from build123d import *

# Parameters (mm, degrees)
SKETCH_1_R      = 1.1
SKETCH_1_R_2    = 1.6
SKETCH_1_R_3    = 15
EXTRUDE_1_DEPTH = 4


with BuildPart() as part:
    # 草图1 → 凸台-拉伸1 (new body)
    with BuildSketch(Plane(origin=(0, 0, 0), x_dir=(1, 0, 0), z_dir=(0, 1, 0))):
        with BuildLine():
            Line((-54, 60), (54, 60))
            ThreePointArc((54, 60), (58.242640687, 58.242640687), (60, 54))
            Line((60, 54), (60, -54))
            ThreePointArc((60, -54), (58.242640687, -58.242640687), (54, -60))
            Line((54, -60), (-54, -60))
            ThreePointArc((-54, -60), (-58.242640687, -58.242640687), (-60, -54))
            Line((-60, -54), (-60, 54))
            ThreePointArc((-60, 54), (-58.242640687, 58.242640687), (-54, 60))
        make_face()
        with Locations(Location((0, 18.6, 0), (0, 0, 270))):
            Circle(SKETCH_1_R, mode=Mode.SUBTRACT)
        with Locations(Location((8.8, -18.6, 0), (0, 0, 270))):
            Circle(SKETCH_1_R, mode=Mode.SUBTRACT)
        with Locations(Location((-8.8, -18.6, 0), (0, 0, 270))):
            Circle(SKETCH_1_R, mode=Mode.SUBTRACT)
        with Locations(Location((-21, 25, 0), (0, 0, 270))):
            Circle(SKETCH_1_R_2, mode=Mode.SUBTRACT)
        with Locations(Location((21, 25, 0), (0, 0, 90))):
            Circle(SKETCH_1_R_2, mode=Mode.SUBTRACT)
        with Locations(Location((21, -25, 0), (0, 0, 270))):
            Circle(SKETCH_1_R_2, mode=Mode.SUBTRACT)
        with Locations(Location((-21, -25, 0), (0, 0, 90))):
            Circle(SKETCH_1_R_2, mode=Mode.SUBTRACT)
        with Locations(Location((-56.25, 50, 0), (0, 0, 270))):
            Circle(SKETCH_1_R_2, mode=Mode.SUBTRACT)
        with Locations(Location((-44.25, 50, 0), (0, 0, 270))):
            Circle(SKETCH_1_R_2, mode=Mode.SUBTRACT)
        with Locations(Location((-44.25, 22, 0), (0, 0, 270))):
            Circle(SKETCH_1_R_2, mode=Mode.SUBTRACT)
        with Locations(Location((-56.25, 22, 0), (0, 0, 270))):
            Circle(SKETCH_1_R_2, mode=Mode.SUBTRACT)
        with Locations(Location((56.25, 22, 0), (0, 0, 270))):
            Circle(SKETCH_1_R_2, mode=Mode.SUBTRACT)
        with Locations(Location((44.25, 22, 0), (0, 0, 270))):
            Circle(SKETCH_1_R_2, mode=Mode.SUBTRACT)
        with Locations(Location((44.25, 50, 0), (0, 0, 270))):
            Circle(SKETCH_1_R_2, mode=Mode.SUBTRACT)
        with Locations(Location((56.25, 50, 0), (0, 0, 270))):
            Circle(SKETCH_1_R_2, mode=Mode.SUBTRACT)
        with Locations(Location((56.25, -50, 0), (0, 0, 270))):
            Circle(SKETCH_1_R_2, mode=Mode.SUBTRACT)
        with Locations(Location((44.25, -50, 0), (0, 0, 270))):
            Circle(SKETCH_1_R_2, mode=Mode.SUBTRACT)
        with Locations(Location((44.25, -22, 0), (0, 0, 270))):
            Circle(SKETCH_1_R_2, mode=Mode.SUBTRACT)
        with Locations(Location((56.25, -22, 0), (0, 0, 270))):
            Circle(SKETCH_1_R_2, mode=Mode.SUBTRACT)
        with Locations(Location((-44.25, -50, 0), (0, 0, 270))):
            Circle(SKETCH_1_R_2, mode=Mode.SUBTRACT)
        with Locations(Location((-56.25, -50, 0), (0, 0, 270))):
            Circle(SKETCH_1_R_2, mode=Mode.SUBTRACT)
        with Locations(Location((-56.25, -22, 0), (0, 0, 270))):
            Circle(SKETCH_1_R_2, mode=Mode.SUBTRACT)
        with Locations(Location((-44.25, -22, 0), (0, 0, 270))):
            Circle(SKETCH_1_R_2, mode=Mode.SUBTRACT)
        with Locations(Location((0, 0, 0), (0, 0, 270))):
            Circle(SKETCH_1_R_3, mode=Mode.SUBTRACT)
        with BuildLine():
            Line((-2, -25), (2, -25))
            ThreePointArc((2, -25), (4.121320344, -25.878679656), (5, -28))
            Line((5, -28), (5, -42))
            ThreePointArc((5, -42), (4.121320344, -44.121320344), (2, -45))
            Line((2, -45), (-2, -45))
            ThreePointArc((-2, -45), (-4.121320344, -44.121320344), (-5, -42))
            Line((-5, -42), (-5, -28))
            ThreePointArc((-5, -28), (-4.121320344, -25.878679656), (-2, -25))
        make_face(mode=Mode.SUBTRACT)
        with BuildLine():
            Line((-45, 2), (-45, -2))
            ThreePointArc((-45, -2), (-44.121320344, -4.121320344), (-42, -5))
            Line((-42, -5), (-28, -5))
            ThreePointArc((-28, -5), (-25.878679656, -4.121320344), (-25, -2))
            Line((-25, -2), (-25, 2))
            ThreePointArc((-25, 2), (-25.878679656, 4.121320344), (-28, 5))
            Line((-28, 5), (-42, 5))
            ThreePointArc((-42, 5), (-44.121320344, 4.121320344), (-45, 2))
        make_face(mode=Mode.SUBTRACT)
        with BuildLine():
            Line((2, 45), (-2, 45))
            ThreePointArc((-2, 45), (-4.121320344, 44.121320344), (-5, 42))
            Line((-5, 42), (-5, 28))
            ThreePointArc((-5, 28), (-4.121320344, 25.878679656), (-2, 25))
            Line((-2, 25), (2, 25))
            ThreePointArc((2, 25), (4.121320344, 25.878679656), (5, 28))
            Line((5, 28), (5, 42))
            ThreePointArc((5, 42), (4.121320344, 44.121320344), (2, 45))
        make_face(mode=Mode.SUBTRACT)
        with BuildLine():
            Line((45, -2), (45, 2))
            ThreePointArc((45, 2), (44.121320344, 4.121320344), (42, 5))
            Line((42, 5), (28, 5))
            ThreePointArc((28, 5), (25.878679656, 4.121320344), (25, 2))
            Line((25, 2), (25, -2))
            ThreePointArc((25, -2), (25.878679656, -4.121320344), (28, -5))
            Line((28, -5), (42, -5))
            ThreePointArc((42, -5), (44.121320344, -4.121320344), (45, -2))
        make_face(mode=Mode.SUBTRACT)
    extrude(amount=EXTRUDE_1_DEPTH)


solid = part.part
Can you work these out from the model? Positions are in its coordinate system, mm. Round coordinates to 2 decimals unless told otherwise and drop trailing zeros. Order: outer loops, then holes, each group sorted by start corner. A loop starts at its lowest first (then second) coordinate and runs counter-clockwise, first axis right, second up. Notation, with made-up numbers: M 10,60 L 47,60 A32 ccw 47,97 Z; hole C 6,1.25 d7. An arc over 180 degrees is marked long. Use a Markdown table: item, result.
1) Imagine slicing it at B-B (x = -33). List the corners of the cut face in (y, z) for me, then the cut area to 3 significant figures.
Geometry says:
| item | result |
|---|---|
| outline | M 0,-60 L 4,-60 L 4,-5 L 0,-5 Z; M 0,5 L 4,5 L 4,60 L 0,60 Z |
| area | 440 mm² |
2) If I drill on line 1 along X through (y, z) = (1.5, -22); line 2 along Z through (x, y) = (-38, 2.9), over which ranges is the centre line in solid material (lowest first)?
Geometry says:
| item | result |
|---|---|
| line 1 | x = -60 to -57.85, -54.65 to -45.85, -42.65 to 42.65, 45.85 to 54.65, 57.85 to 60 |
| line 2 | z = -60 to -5, 5 to 60 |
3) Imagine slicing it at C-C (z = -22). List the corners of the cut face in (x, y) for me.
Geometry says:
| item | result |
|---|---|
| outline | M -60,0 L -57.85,0 L -57.85,4 L -60,4 Z; M -54.65,0 L -45.85,0 L -45.85,4 L -54.65,4 Z; M -42.65,0 L 42.65,0 L 42.65,4 L -42.65,4 Z; M 45.85,0 L 54.65,0 L 54.65,4 L 45.85,4 Z; M 57.85,0 L 60,0 L 60,4 L 57.85,4 Z |
4) If we mould it in two halves opening along Z, with no side actions, what happens to faces 1 (the face through (-5, 2, -35)), 2 (the face through (1, 2, 60)), 3 (the face through (-19.414, 1.972, -25.208))? For each: +Z half, -Z half, draft (parallel to the pull), parting line (faces both ways), or undercut.
Geometry says:
| item | result |
|---|---|
| face 1 | undercut |
| face 2 | +Z half |
| face 3 | undercut |
5) Imagine slicing it at D-D (z = -40.5). List the corners of the cut face in (x, y) for me, then the cut area to 3 significant figures.
Geometry says:
| item | result |
|---|---|
| outline | M -60,0 L -5,0 L -5,4 L -60,4 Z; M 5,0 L 60,0 L 60,4 L 5,4 Z |
| area | 440 mm² |
6) Imagine slicing it at A-A (z = 0). List the corners of the cut face in (x, y) for me, then the cut area to 3 significant figures.
Geometry says:
| item | result |
|---|---|
| outline | M -60,0 L -45,0 L -45,4 L -60,4 Z; M -25,0 L -15,0 L -15,4 L -25,4 Z; M 15,0 L 25,0 L 25,4 L 15,4 Z; M 45,0 L 60,0 L 60,4 L 45,4 Z |
| area | 200 mm² |
